Here's the drawing with two shaded views (mm, measured from the low corner). I have some questions. Coordinates: 2 decimals unless noted, no trailing zeros. Write each loop counter-clockwise with the first axis right and the second up, starting at its lowest first coordinate (ties: lowest second). Pieces come first, ordered by that corner, then holes. Notation, with made-up numbers: (1.5, -13) -> (55.5, -13) arc R24 cw to (55.5, 23) -> close; hole circle Ø1 at (-31, 62). An arc over 180 degrees is marked (long way). Use one line per item in the form item = value.
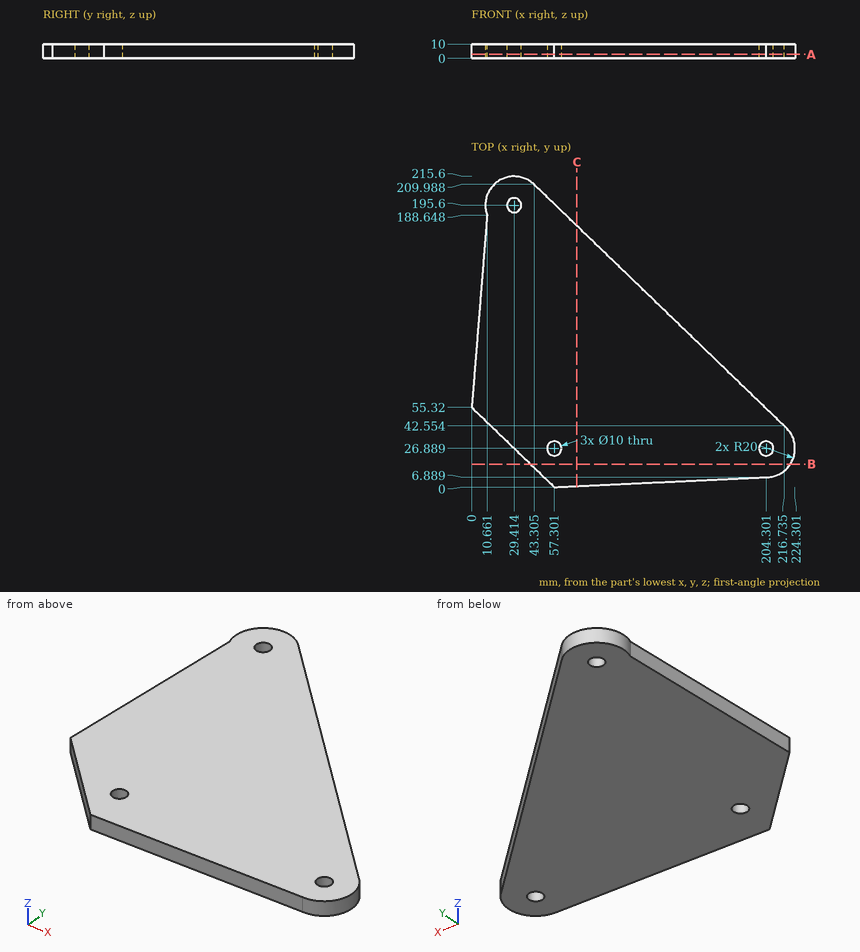
Q1. If I drill on line 1 (Y direction, x = 169.5, z = 1) (1 decimal); line 2 (Y direction, x = 59, z = 6) (1 decimal); line 3 (Y direction, x = 18, z = 4.5) (1 decimal), over which ranges is the centre line in solid material (lowest first)? Write a range as from..to.
Return value:
line_1 = 5.3..88.2
line_2 = 0.1..22.2, 31.6..194.8
line_3 = 37.9..212
Q2. Will these pins go through, and if not, where does the flat tip stop? pin 1 (5 mm diameter, centred on y = 77.5, z = 4.5, fed in from -X); pin 2 (1.5 mm diameter, centred on y = 113, z = 4, fed in from -X); pin 3 (1.5 mm diameter, centred on x = 171, z = 5, fed in from +Y); pin 4 (11.5 mm diameter, centred on x = 57.3, y = 26.89, fed in from +Z).
Return value:
pin_1 = 1.57
pin_2 = 4.55
pin_3 = 87.43
pin_4 = 10
Q3. Suppose I cut it at A-A (z = 2.75). Write out the boundary of the cut face in (x, y) (1 decimal).
Return value:
outline = (0, 55.3) -> (57.3, 0) -> (204.3, 6.9) arc R20 ccw to (216.7, 42.6) -> (43.3, 210) arc R20 ccw to (10.7, 188.6) -> close; hole circle Ø10 at (29.4, 195.6); hole circle Ø10 at (57.3, 26.9); hole circle Ø10 at (204.3, 26.9)
Q4. Suppose I cut it at C-C (x = 73). Write out the boundary of the cut face in (y, z) (1 decimal), then the cut area to 3 significant figures.
Return value:
outline = (0.7, 0) -> (181.3, 0) -> (181.3, 10) -> (0.7, 10) -> close
area = 1,810 mm2
Q5. Suppose I cut it at B-B (y = 16). Write out the boundary of the cut face in (x, z), then the cut area to 3 significant figures.
Return value:
outline = (40.73, 0) -> (221.08, 0) -> (221.08, 10) -> (40.73, 10) -> close
area = 1,800 mm2
